```python
from build123d import *

# Parameters (mm, degrees)
SKETCH1_R           = 25
BOSS_EXTRUDE2_DEPTH = 210
SKETCH2_R           = 15
BOSS_EXTRUDE3_DEPTH = 1
SKETCH3_R           = 7.5
BOSS_EXTRUDE4_DEPTH = 2
SKETCH4_R           = 6
BOSS_EXTRUDE5_DEPTH = 25


with BuildPart() as part:
    # Sketch1 → Boss-Extrude2 (new body)
    with BuildSketch(Plane.XY):
        Circle(SKETCH1_R)
    extrude(amount=-BOSS_EXTRUDE2_DEPTH)

    # Sketch2 → Boss-Extrude3 (add)
    with BuildSketch(Plane.XY):
        Circle(SKETCH2_R)
    extrude(amount=BOSS_EXTRUDE3_DEPTH)

    # Sketch3 → Boss-Extrude4 (add)
    with BuildSketch(Plane.XY.offset(1)):
        Circle(SKETCH3_R)
    extrude(amount=BOSS_EXTRUDE4_DEPTH)

    # Sketch4 → Boss-Extrude5 (add)
    with BuildSketch(Plane.XY.offset(3)):
        Circle(SKETCH4_R)
    extrude(amount=BOSS_EXTRUDE5_DEPTH)


solid = part.part
```
Input: part model. Units: mm. Frame: model coordinates. A direction names the side the tool comes from. Coordinates: 2 decimals unless noted, no trailing zeros. Loops run counter-clockwise (first coordinate to the right, second up) from the corner with the lowest first, then second, coordinate; pieces in that order, holes last.
Q1. Set-up query: faces 1 (the cylindrical face through (23.846, 7.509, -103.53)), 2 (the cylindrical face through (-7.493, 0.33, 1.986)). Return all of +Z, -Z, +X, -X, +Y, -Y with unobstructed straight access to the full face (end or side cutting, diameter ignored); none if empty.
Results are:
face 1: +Z, -Z
face 2: +Z
Q2. Section C-C, the plane z = -161. Return the cut outline in (x, y), and give its area (3 significant figures).
Results are:
outline: circle Ø50 at (0, 0)
area: 1,960 mm2
Q3. Contact query for flat-ended pins moving along their axis: pin 1 (4 mm diameter, centred on x = 12.5, z = -98, fed in from +Y); pin 2 (8 mm diameter, centred on x = -5, z = -123.5, fed in from -Y); pin 3 (4 mm diameter, centred on x = 5.5, z = -114, fed in from -Y). Output: stop coordinate, or through.
Results are:
pin 1: stops at y = 22.69
pin 2: stops at y = -24.98
pin 3: stops at y = -24.75
Q4. Section A-A, the plane y = 0. Return the cut outline in (x, z), and give its area (3 significant figures).
Results are:
outline: (-25, -210) - (25, -210) - (25, 0) - (15, 0) - (15, 1) - (7.5, 1) - (7.5, 3) - (6, 3) - (6, 28) - (-6, 28) - (-6, 3) - (-7.5, 3) - (-7.5, 1) - (-15, 1) - (-15, 0) - (-25, 0) - close
area: 10,900 mm2
Q5. Section D-D, the plane x = -12. Return the cut outline in (y, z).
Results are:
outline: (-21.93, -210) - (21.93, -210) - (21.93, 0) - (9, 0) - (9, 1) - (-9, 1) - (-9, 0) - (-21.93, 0) - close
Q6. Line query: line 1 along Z through (x, y) = (12, 9.5); line 2 along X through (y, z) = (-0.5, -76.5) (3 decimals); line 3 along Z through (x, y) = (-10, 10). Output: solid intervals per line, ascending.
Results are:
line 1: z = -210 to 0
line 2: x = -24.995 to 24.995
line 3: z = -210 to 1
